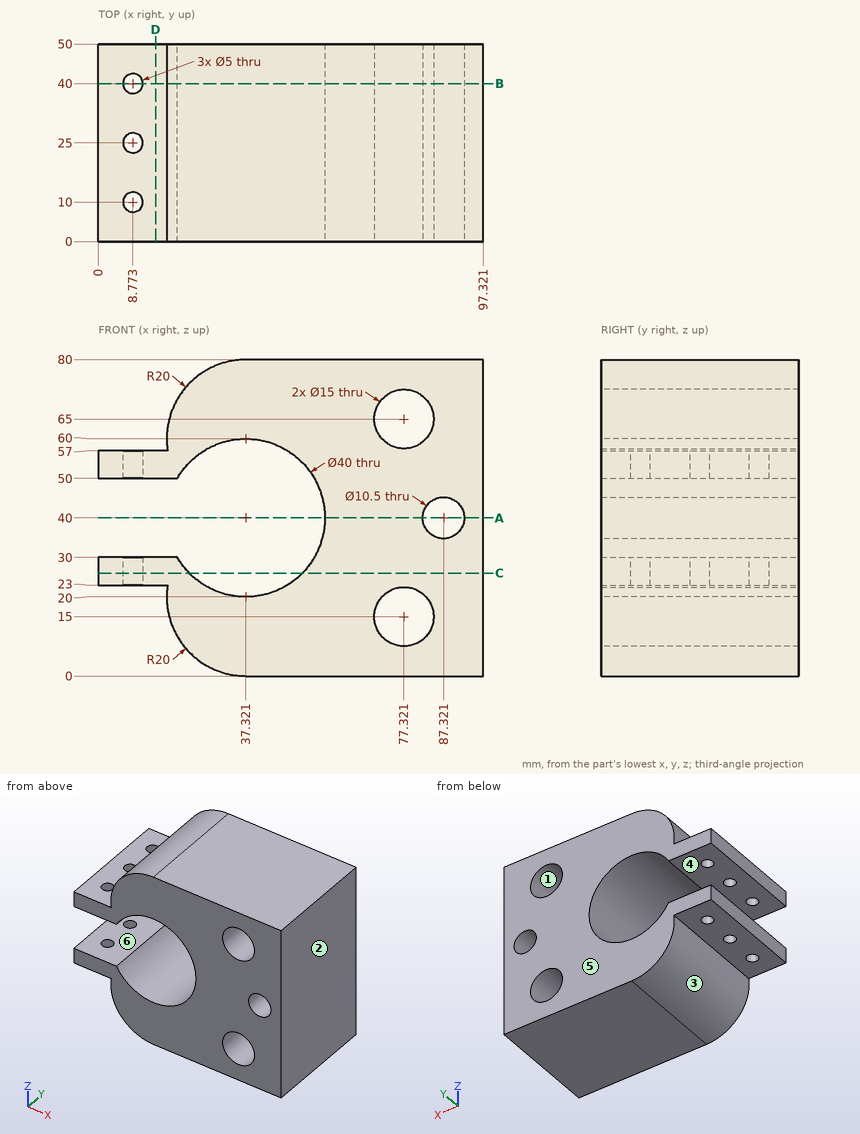
Study the drawing (mm; zero at the part's minimum x, y, z) and answer. A direction names the side the tool comes from. Give positions to 0.01 mm unless a question says otherwise; leave off trailing zeros. Loops run counter-clockwise (first coordinate to the right, second up) from the corner with the lowest first, then second, coordinate; pieces in that order, holes last. Notation, with made-up numbers: (56.5, 55.5) - (95.5, 55.5) arc R23 cw to (95.5, 73.5) - close; hole circle Ø10 at (44.5, 51.25). An arc over 180 degrees is marked (long way). Answer in a Markdown table with one row per item. Add a question column.
Q1. A tool of negligible diameter and unlimited length cuts with its end or side. For the marked faces 5 and 6, from which of +Z, -Z, +X, -X, +Y, -Y can it reach the whole face along a straight path? Write none if from no direction.
Q2. The part is cut by section D-D (x = 14.5). Determine the outline of the cut face in (y, z).
Q3. The part is cut by section B-B (y = 40). Determine the outline of the cut face in (x, z).
Q4. Consider line 1 along Z through (x, y) = (77.5, 38); line 2 along Z through (x, y) = (73, 11.5); line 3 along Z through (x, y) = (6, 46). Determine where each line is inside the solid, lowest interval first.
Q5. Each of these flat-tipped pins is pushed along its axis until it touches: P1, Ø6.5, axis at x = 8.77, y = 40, coming from the -Z side; P2, Ø19.5, axis at x = 13, y = 23, coming from the +Z side; P3, Ø19.5, axis at x = 10, y = 18.5, coming from the -Z side (1 decimal). Where does it stop, or does it pass through?
Q6. Determine the mould class of the marked faces 1, 2, 3 and 4 for opening direction X: released by +X, released by -X, zero draft, split by the parting line, or undercut.
Q7. The part is cut by section A-A (z = 40). Determine the outline of the cut face in (x, y), and give its area (4 significant figures).
Q8. The part is cut by section C-C (z = 26). Determine the outline of the cut face in (x, y).
Solution:
| question | item | result |
|---|---|---|
| 1 | face 5 | +Z, -Z, +X, -X, +Y |
| 1 | face 6 | -X, +Y, -Y |
| 2 | outline | (0, 23) - (50, 23) - (50, 30) - (0, 30) - close; (0, 50) - (50, 50) - (50, 57) - (0, 57) - close |
| 3 | outline | (0, 23) - (6.27, 23) - (6.27, 30) - (0, 30) - close; (0, 50) - (6.27, 50) - (6.27, 57) - (0, 57) - close; (11.27, 23) - (17.55, 23) arc R20 ccw to (37.32, 0) - (97.32, 0) - (97.32, 80) - (37.32, 80) arc R20 ccw to (17.55, 57) - (11.27, 57) - (11.27, 50) - (20, 50) arc R20 cw (long way) to (20, 30) - (11.27, 30) - close; hole circle Ø15 at (77.32, 15); hole circle Ø15 at (77.32, 65); hole circle Ø10.5 at (87.32, 40) |
| 4 | line 1 | z = 0 to 7.5, 22.5 to 57.5, 72.5 to 80 |
| 4 | line 2 | z = 0 to 8.87, 21.13 to 58.87, 71.13 to 80 |
| 4 | line 3 | z = 23 to 30, 50 to 57 |
| 5 | P1 | stops at z = 23 |
| 5 | P2 | stops at z = 73.7 |
| 5 | P3 | stops at z = 10.4 |
| 6 | face 1 | undercut |
| 6 | face 2 | released by +X |
| 6 | face 3 | released by -X |
| 6 | face 4 | zero draft |
| 7 | outline | (57.32, 0) - (82.07, 0) - (82.07, 50) - (57.32, 50) - close; (92.57, 0) - (97.32, 0) - (97.32, 50) - (92.57, 50) - close |
| 7 | area | 1,475 mm² |
| 8 | outline | (0, 0) - (23.04, 0) - (23.04, 50) - (0, 50) - close; (51.6, 0) - (97.32, 0) - (97.32, 50) - (51.6, 50) - close; hole circle Ø5 at (8.77, 10); hole circle Ø5 at (8.77, 25); hole circle Ø5 at (8.77, 40) |
